For this review, take the finished solid that the model builds, in its own axes (mm). Face numbers are marked on the shaded views. A direction names the side the tool comes from. Round coordinates to 2 decimals unless told otherwise and drop trailing zeros. Loops run counter-clockwise (first coordinate to the right, second up) from the corner with the lowest first, then second, coordinate; pieces in that order, holes last. Notation, with made-up numbers: (67.5, -4.5) -> (113.5, -4.5) arc R17 ccw to (113.5, 8.5) -> close; hole circle Ø7 at (-38.5, 78.25). An arc over 180 degrees is marked (long way). Use one line per item in the form item = value. Start each with the question number.
from build123d import *

# Parameters (mm, degrees)
SKETCH2_R           = 3
BOSS_EXTRUDE1_DEPTH = 20


with BuildPart() as part:
    # Sketch1 → Revolve1 (revolve)
    with BuildSketch(Plane.XY):
        Polygon((0, 0), (10, 0), (10, 1), (5, 1), (5, 4), (10, 4), (10, 5), (0, 5), align=None)
    revolve(axis=Axis((0, 5, 0), (0, -1, 0)))

    # Sketch2 → Boss-Extrude1 (add)
    with BuildSketch(Plane(origin=(0, 5, 0), x_dir=(1, 0, 0), z_dir=(0, 1, 0))):
        Circle(SKETCH2_R)
    extrude(amount=BOSS_EXTRUDE1_DEPTH)


solid = part.part
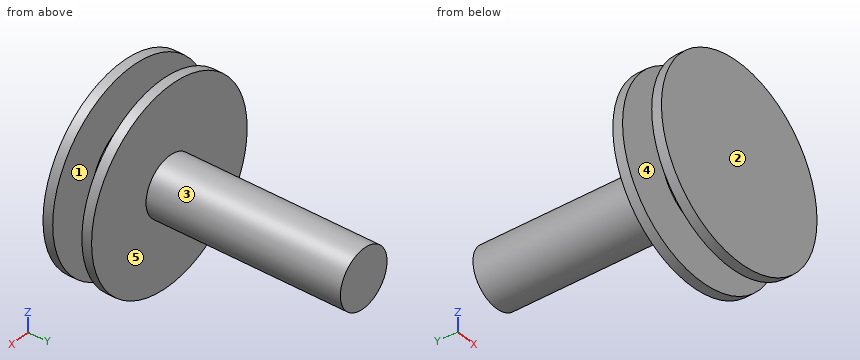
Item 1: Wall thickness on line 1 (Y direction, x = 6.75, z = 1); line 2 (Z direction, x = 0, y = 15.5); line 3 (Z direction, x = -1.75, y = 20): over which ranges is each line inside the solid? List them lowest first.
Item 2: Machinability: for the marked faces 1 and 2, which of the approach directions +Z, -Z, +X, -X, +Y, -Y give a long, thin tool a straight path to every point of the face, cutting with its end or side? Answer none if there is none.
Item 3: Take a section at B-B on z = 7.5. Give the boundary of the cut face in (x, y).
Item 4: For P1, Ø5, axis at y = 8.5, z = 0.5, coming from the +X side; P2, Ø12, axis at x = 6.5, y = 3, coming from the -Z side; P3, Ø6, axis at x = -0.5, y = 20.5, coming from the -Z side, all flat-tipped, find the tip position at first contact; note any pin that passes through.
Item 5: Take a section at D-D on z = -1.5. Give the boundary of the cut face in (x, y), plus the area to 3 significant figures.
Item 6: Take a section at A-A on x = 6. Give the boundary of the cut face in (y, z), plus the area to 3 significant figures.
Item 7: Draft analysis for pull direction Y (two halves, no side actions). For the marked faces 3, 4 and 5, state which applies: +Y half, -Y half, draft (parallel to the pull), parting line (faces both ways), or undercut.
Item 8: Take a section at C-C on x = 0. Give the boundary of the cut face in (y, z), plus the area to 3 significant figures.
Results:
q1.line_1 = 0 to 1, 4 to 5
q1.line_2 = -3 to 3
q1.line_3 = -2.44 to 2.44
q2.face_1 = none
q2.face_2 = +Z, -Z, +X, -X, -Y
q3.outline = (-6.61, 0) -> (6.61, 0) -> (6.61, 1) -> (-6.61, 1) -> close; (-6.61, 4) -> (6.61, 4) -> (6.61, 5) -> (-6.61, 5) -> close
q4.P1 = 3
q4.P2 = -9.98
q4.P3 = -3
q5.outline = (-9.89, 0) -> (9.89, 0) -> (9.89, 1) -> (4.77, 1) -> (4.77, 4) -> (9.89, 4) -> (9.89, 5) -> (2.6, 5) -> (2.6, 25) -> (-2.6, 25) -> (-2.6, 5) -> (-9.89, 5) -> (-9.89, 4) -> (-4.77, 4) -> (-4.77, 1) -> (-9.89, 1) -> close
q5.area = 172 mm2
q6.outline = (0, -8) -> (1, -8) -> (1, 8) -> (0, 8) -> close; (4, -8) -> (5, -8) -> (5, 8) -> (4, 8) -> close
q6.area = 32.0 mm2
q7.face_3 = draft
q7.face_4 = undercut
q7.face_5 = +Y half
q8.outline = (0, -10) -> (1, -10) -> (1, -5) -> (4, -5) -> (4, -10) -> (5, -10) -> (5, -3) -> (25, -3) -> (25, 3) -> (5, 3) -> (5, 10) -> (4, 10) -> (4, 5) -> (1, 5) -> (1, 10) -> (0, 10) -> close
q8.area = 190 mm2
